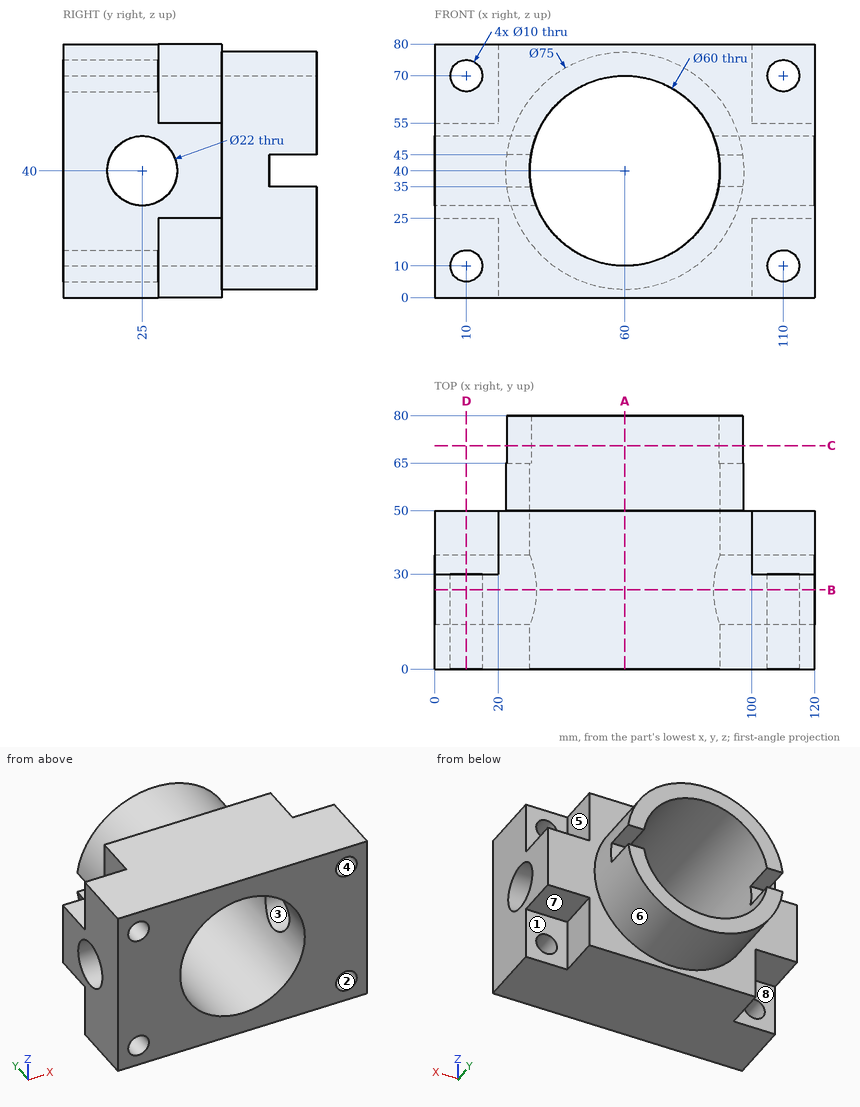
Answer from the drawing. Dimensions are ordinates in mm from the lowest x, y and z of the part. A direction names the side the tool comes from. Round coordinates to 2 decimals unless told otherwise and drop trailing zeros. Loops run counter-clockwise (first coordinate to the right, second up) from the corner with the lowest first, then second, coordinate; pieces in that order, holes last. Notation, with made-up numbers: M 31,82 L 44,82 A21 cw 44,100 Z; hole C 17,-16.5 d10. An arc over 180 degrees is marked long. One line per question, with ' | ' between items. Start each with the question number.
(1) A cutting plane is placed at B-B on y = 25. Write down the section's boundary in (x, z).
(2) A cutting plane is placed at D-D on x = 10. Write down the section's boundary in (y, z).
(3) Flat-ended cylindrical pins translate along their axes: pin 1 Ø2.5 at (x, y) = (27, 76) entering from -Z; pin 2 Ø22 at (x, z) = (11.5, 13) entering from +Y; pin 3 Ø10 at (y, z) = (41.5, 66.5) entering from +X; pin 4 Ø3 at (x, y) = (22.5, 50.5) entering from -Z. Find the tip coordinate at first contact, or state that the pin passes through.
(4) Find the intervals of material crossed by line 1 (Z direction, x = 10, y = 13); line 2 (Z direction, x = 59, y = 73.5); line 3 (X direction, y = 13.5, z = 14), in increasing order.
(5) A cutting plane is placed at C-C on y = 70.5. Write down the section's boundary in (x, z), plus the area to 3 significant figures.
(6) A tool of negligible diameter and unlimited length cuts with its end or side. For the marked faces 4, 5, 6, 7 and 8, from which of +Z, -Z, +X, -X, +Y, -Y can it reach the whole face along a straight path? Write none if from no direction.
(7) For a pull along Y with two mould halves and no side action, classify the marked faces 1, 2 and 3 as released by +Y, released by -Y, zero draft, split by the parting line, or undercut.
(8) A cutting plane is placed at A-A on x = 60. Write down the section's boundary in (y, z).
Geometry check:
1) outline: M 0,0 L 120,0 L 120,29 L 87.91,29 A30 cw 32.09,29 L 0,29 Z; M 0,51 L 32.09,51 A30 cw 87.91,51 L 120,51 L 120,80 L 0,80 Z; hole C 10,10 d10; hole C 10,70 d10; hole C 110,10 d10; hole C 110,70 d10
2) outline: M 0,0 L 30,0 L 30,5 L 0,5 Z; M 0,15 L 30,15 L 30,25 L 50,25 L 50,55 L 30,55 L 30,65 L 0,65 Z; M 0,75 L 30,75 L 30,80 L 0,80 Z; hole C 25,40 d22
3) pin 1: stops at z = 20.05 | pin 2: stops at y = 50 | pin 3: stops at x = 100 | pin 4: stops at z = 0
4) line 1: z = 0 to 5, 15 to 65, 75 to 80 | line 2: z = 2.51 to 10.02, 69.98 to 77.49 | line 3: x = 0 to 7, 13 to 45.03, 74.97 to 107, 113 to 120
5) outline: M 22.83,35 A37.5 ccw 97.17,35 L 89.58,35 A30 cw 30.42,35 Z; M 22.83,45 L 30.42,45 A30 cw 89.58,45 L 97.17,45 A37.5 ccw Z | area: 1,440 mm²
6) face 4: +Y, -Y | face 5: +Z, +X, +Y | face 6: +Y | face 7: -Z, +X, +Y | face 8: -Z, -X, +Y
7) face 1: released by +Y | face 2: zero draft | face 3: undercut
8) outline: M 0,0 L 50,0 L 50,2.5 L 80,2.5 L 80,10 L 0,10 Z; M 0,70 L 80,70 L 80,77.5 L 50,77.5 L 50,80 L 0,80 Z
